Check sheet for the modelled part. Datum: model origin and axes. Units: mm. A direction names the side the tool comes from. Coordinates: 2 decimals unless noted, no trailing zeros. Write each loop counter-clockwise with the first axis right and the second up, starting at its lowest first coordinate (ties: lowest second). Pieces come first, ordered by that corner, then holes. Notation, with made-up numbers: (-4, -12.75) -> (45, -12.75) arc R21 ccw to (45, -1.75) -> close; hole circle Ø7 at (32.5, 22.5). An arc over 180 degrees is marked (long way). One line per item, written item: value. Start each with the question number.
1) Draft check along X on faces 1 (the flat face through (42, -2, -30)), 2 (the flat face through (27.263, -1.578, 19.157)), 3 (the cylindrical face through (13.16, -1.58, -58.31)). Enter one of: +X half, -X half, draft (parallel to the pull), parting line (faces both ways), or undercut.
2) Scan lines: line 1 along Z through (x, y) = (0, -1.4); line 2 along Z through (x, y) = (40.5, -0.55); line 3 along X through (y, z) = (-1.6, -58). Record each from-to range of solid material in increasing order. Write a range as [from, to].
3) Set-up check for faces 4 (the flat face through (-31.743, -1.578, -12.202)), 5 (the flat face through (37.183, -1.578, -50.28)), 6 (the flat face through (38, -2, -5)): record each of +Z, -Z, +X, -X, +Y, -Y from which the full face is reachable in a straight line by a thin tool's end or side.
4) Gauge pin test, flat end, axial feed: P1, Ø5, axis at x = 33.29, z = -23, coming from the +Y side. Record the tip position at first contact, or that the pin passes through.
5) Sectioned sample at C-C on z = -60. Enter the section's corners in (x, y).
6) Sectioned sample at B-B on y = -2.05. Enter the section's corners in (x, z), plus the area to 3 significant figures.
7) Sectioned sample at D-D on z = -23. Enter the section's corners in (x, y), plus the area to 3 significant figures.
8) Sectioned sample at A-A on x = 0. Enter the section's corners in (y, z).
```python
from build123d import *

# Parameters (mm, degrees)
F0_R     = 2.5
F0_R_2   = 1.5
F0_R_3   = 4.5
F1_DEPTH = 3.2
F2_R     = 5


with BuildPart() as f1:
    # F0 (on Front) → F1 (new body)
    with BuildSketch(Plane.XZ):
        with BuildLine():
            Line((-23.714286, 44), (-40, -70))
            Line((-40, -70), (40, -70))
            Line((40, -70), (34.285714, -30))
            Line((34.285714, -30), (50.285714, -30))
            Line((50.285714, -30), (50.285714, -5))
            Line((50.285714, -5), (30.714286, -5))
            Line((30.714286, -5), (23.714286, 44))
            ThreePointArc((23.714286, 44), (0, 67.714286), (-23.714286, 44))
        make_face()
        with Locations((-15, -60)):
            Circle(F0_R, mode=Mode.SUBTRACT)
        with Locations((15, -60)):
            Circle(F0_R, mode=Mode.SUBTRACT)
        with Locations((33.285714, -23)):
            Circle(F0_R_2, mode=Mode.SUBTRACT)
        with Locations((0, 44)):
            Circle(F0_R_3, mode=Mode.SUBTRACT)
    extrude(amount=F1_DEPTH)

    # F2
    f2_edges = [f1.edges().sort_by_distance(p)[0] for p in [
        (50.285714, -1.6, -5),
    ]]
    fillet(f2_edges, radius=F2_R)


solid = f1.part
```
Answers:
1. face 1: draft
1. face 2: +X half
1. face 3: undercut
2. line 1: z = [-70, 39.5], [48.5, 67.71]
2. line 2: z = [-30, -5]
2. line 3: x = [-38.29, -16.5], [-13.5, 13.5], [16.5, 38.29]
3. face 4: +Z, -X, +Y, -Y
3. face 5: +X, +Y, -Y
3. face 6: +Z, +X, +Y, -Y
4. P1: stops at y = 0
5. outline: (-38.57, -3.2) -> (-17.5, -3.2) -> (-17.5, 0) -> (-38.57, 0) -> close; (-12.5, -3.2) -> (12.5, -3.2) -> (12.5, 0) -> (-12.5, 0) -> close; (17.5, -3.2) -> (38.57, -3.2) -> (38.57, 0) -> (17.5, 0) -> close
6. outline: (-40, -70) -> (40, -70) -> (34.29, -30) -> (50.29, -30) -> (50.29, -10) arc R5 ccw to (45.29, -5) -> (30.71, -5) -> (23.71, 44) arc R23.71 ccw to (-23.71, 44) -> close; hole circle Ø5 at (-15, -60); hole circle Ø9 at (0, 44); hole circle Ø5 at (15, -60); hole circle Ø3 at (33.29, -23)
6. area: 8,480 mm2
7. outline: (-33.29, -3.2) -> (31.79, -3.2) -> (31.79, 0) -> (-33.29, 0) -> close; (34.79, -3.2) -> (50.29, -3.2) -> (50.29, 0) -> (34.79, 0) -> close
7. area: 258 mm2
8. outline: (-3.2, -70) -> (0, -70) -> (0, 39.5) -> (-3.2, 39.5) -> close; (-3.2, 48.5) -> (0, 48.5) -> (0, 67.71) -> (-3.2, 67.71) -> close
